Geometry: final body of the model. Coordinates: model frame, mm. Face numbers are marked on the shaded views. A direction names the side the tool comes from. Coordinates: 2 decimals unless noted, no trailing zeros. Order: outer loops, then holes, each group sorted by start corner. A loop starts at its lowest first (then second) coordinate and runs counter-clockwise, first axis right, second up. Notation, with made-up numbers: (22.5, -33) - (78.5, -33) arc R19 cw to (78.5, -3) - close; hole circle Ø4 at (-27.5, 64.5). An arc over 180 degrees is marked (long way). Use a Markdown table: item, result. Add a question column.
```python
from build123d import *

# Parameters (mm, degrees)
F2_DEPTH = 7.92
F3_R     = 0.5
F5_R     = 1.968691
F6_DEPTH = 1


with BuildPart() as f2:
    # F1 (on Top) → F2 (new body)
    with BuildSketch(Plane.XY):
        with BuildLine():
            Line((-5.330044, 4.538535), (-9.425229, 4.688782))
            ThreePointArc((-9.425229, 4.688782), (0, -10.527089), (9.425229, 4.688782))
            Line((9.425229, 4.688782), (5.330044, 4.538535))
            ThreePointArc((5.330044, 4.538535), (0, -7.000548), (-5.330044, 4.538535))
        make_face()
    extrude(amount=F2_DEPTH)

    # F3
    f3_edges = [f2.edges().sort_by_distance(p)[0] for p in [
        (-5.330044, 4.538535, 3.96),
        (5.330044, 4.538535, 3.96),
    ]]
    fillet(f3_edges, radius=F3_R)

    # F5 (on offset) → F6 (cut)
    with BuildSketch(Plane.XZ.offset(10.5)):
        with Locations((0.012802, 4.007582)):
            Circle(F5_R)
    extrude(amount=-F6_DEPTH, mode=Mode.SUBTRACT)


solid = f2.part
```
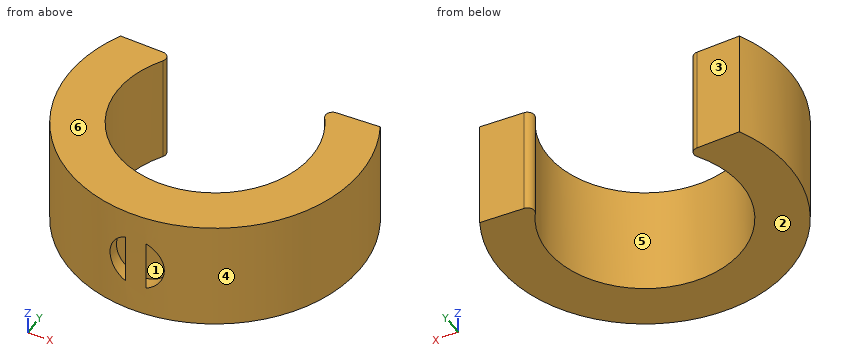
1) Pin query (flat end, axial travel): pin 1 (2 mm diameter, centred on y = -6.5, z = 4.5, fed in from +X); pin 2 (1.5 mm diameter, centred on x = 1.5, z = 5.5, fed in from +Y); pin 3 (4 mm diameter, centred on y = -4, z = 2.5, fed in from +X). Return the tip coordinate at first contact, or that it passes through.
2) Ray query, line 1 along X through (y, z) = (0.25, 4); line 2 along Z through (x, y) = (-1.75, -10); line 3 along X through (y, z) = (-4.5, 4). Return the intervals inside material, ascending.
3) Section C-C (y = -5.5). Return loops of the section in (x, z), then the cut area to 3 significant figures.
4) Draft query along X for the marked faces 4, 5 and 6. Return one class per face: pulls with the +X half, pulls with the -X half, needs draft (parallel to the pull), parting line crosses it, or undercut.
5) Set-up query: the marked faces 1, 2 and 3. Return all of +Z, -Z, +X, -X, +Y, -Y with unobstructed straight access to the full face (end or side cutting, diameter ignored); none if empty.
6) Section B-B (x = 1.5). Return loops of the section in (y, z), then the cut area to 3 significant figures.
7) Section D-D (z = 6.25). Return loops of the section in (x, y), then the cut area to 3 significant figures.
8) Section A-A (y = 0). Return loops of the section in (x, z), then the cut area to 3 significant figures.
Values follow:
| question | item | result |
|---|---|---|
| 1 | pin 1 | stops at x = 8.98 |
| 1 | pin 2 | stops at y = -6.63 |
| 1 | pin 3 | stops at x = 10.34 |
| 2 | line 1 | x = -10.52 to -7, 7 to 10.52 |
| 2 | line 2 | z = 0 to 3.13, 4.88 to 7.92 |
| 2 | line 3 | x = -9.52 to -5.36, 5.36 to 9.52 |
| 3 | outline | (-8.98, 0) - (-4.33, 0) - (-4.33, 7.92) - (-8.98, 7.92) - close; (4.33, 0) - (8.98, 0) - (8.98, 7.92) - (4.33, 7.92) - close |
| 3 | area | 73.6 mm² |
| 4 | face 4 | parting line crosses it |
| 4 | face 5 | undercut |
| 4 | face 6 | needs draft |
| 5 | face 1 | none |
| 5 | face 2 | -Z, +X, -X, +Y, -Y |
| 5 | face 3 | +Z, -Z, +Y |
| 6 | outline | (-10.42, 0) - (-6.84, 0) - (-6.84, 7.92) - (-10.42, 7.92) - (-10.42, 5.3) - (-9.5, 5.3) - (-9.5, 2.72) - (-10.42, 2.72) - close |
| 6 | area | 26.0 mm² |
| 7 | outline | (-9.43, 4.69) arc R10.53 ccw (long way) to (9.43, 4.69) - (6.28, 4.57) arc R0.5 ccw to (5.88, 3.8) arc R7 cw (long way) to (-5.88, 3.8) arc R0.5 ccw to (-6.28, 4.57) - close |
| 7 | area | 131 mm² |
| 8 | outline | (-10.53, 0) - (-7, 0) - (-7, 7.92) - (-10.53, 7.92) - close; (7, 0) - (10.53, 0) - (10.53, 7.92) - (7, 7.92) - close |
| 8 | area | 55.9 mm² |
